Part model, mm, in its own coordinate system. A direction names the side the tool comes from. Give positions to 0.01 mm unless a question says otherwise; leave off trailing zeros. Order: outer loops, then holes, each group sorted by start corner. A loop starts at its lowest first (then second) coordinate and runs counter-clockwise, first axis right, second up.
1. Slice it at B-B on z = 36.5. List the corners of the cut face in (x, y) (3 decimals), and give its area (3 significant figures).
2. Drop flat-ended pins along their axis: pin 1 Ø11 at (x, y) = (5, 8) entering from +Z; pin 2 Ø6.5 at (x, y) = (24.5, 13.5) entering from +Z; pin 3 Ø1 at (x, z) = (-18, 8.5) entering from -Y. Give the stop position or say it passes through.
3. Probe line 1 (X direction, y = -8, z = 11); line 2 (Y direction, x = -13, z = 31); line 3 (X direction, y = 17.5, z = 23). List the from-to ranges inside material, lowest first.
4. Mould opens along X. For faces 1 (the flat face through (-4, 8, 25)), 2 (the flat face through (-35.965, -2.794, 25.832)), 3 (the flat face through (-38.5, 6, 15)) say: +X half, -X half, draft (parallel to the pull), parting line (faces both ways), or undercut.
5. Slice it at D-D on z = 4. List the corners of the cut face in (x, y).
6. Which spindle directions (+Z, -Z, +X, -X, +Y, -Y) get a long thin tool onto all of the face, cutting with end or side? Do faces 4 (the flat face through (22, 10, 35)), 5 (the flat face through (-16, 13, 20)), 6 (the flat face through (1.5, -19, 2)). Say none if no direction does.
7. Slice it at A-A on x = 6.5. List the corners of the cut face in (y, z), and give its area (3 significant figures).
8. Slice it at C-C on y = -18. List the corners of the cut face in (x, z).
from build123d import *

# Parameters (mm, degrees)
F0_W      = 35
F0_H      = 10
F1_DEPTH  = 5
F2_DEPTH  = 10
F3_DEPTH  = 15
F4_DEPTH  = 38
F5_DEPTH  = 38
F7_DEPTH  = 5
F8_DEPTH  = 15
F0_W_2    = 10
F0_H_2    = 22
F9_DEPTH  = 25
F10_DEPTH = 30
F11_DEPTH = 35
F12_DEPTH = 20
F0_W_3    = 5
F0_H_3    = 27
F13_DEPTH = 38


with BuildPart() as f1:
    # F0 (on Top) → F1 (new body)
    with BuildSketch(Plane.XY):
        with Locations((-16, -18.5)):
            Rectangle(F0_W, F0_H)
    extrude(amount=F1_DEPTH)

    # F0 (on Top) → F2 (join)
    with BuildSketch(Plane.XY):
        Polygon((33.5, -13.5), (33.5, -3.5), (11.5, -3.5), (1.5, -3.5), (-8.5, -3.5), (-33.5, -3.5), (-33.5, -13.5), (1.5, -13.5), align=None)
    extrude(amount=F2_DEPTH)

    # F0 (on Top) → F3 (join)
    with BuildSketch(Plane.XY):
        Polygon((38.5, -3.5), (33.5, -3.5), (33.5, -13.5), (33.5, -23.5), (38.5, -23.5), align=None)
    extrude(amount=F3_DEPTH)



with BuildPart() as f4:
    # F0 (on Top) → F4 (new body)
    with BuildSketch(Plane.XY):
        Polygon((11.5, 23.5), (-38.5, 23.5), (-38.5, 18.5), (-33.5, 18.5), (-8.5, 18.5), (1.5, 18.5), (11.5, 18.5), align=None)
    extrude(amount=F4_DEPTH)


with BuildPart() as f1_1:
    add(f1.part)

    add(f4.part)  # F5 merges F4
    # F0 (on Top) → F5 (join)
    with BuildSketch(Plane.XY):
        Polygon((-33.5, 18.5), (-38.5, 18.5), (-38.5, -23.5), (-33.5, -23.5), (-33.5, -13.5), (-33.5, -3.5), align=None)
    extrude(amount=F5_DEPTH)

    # F6 (on face) → F7 (cut)
    with BuildSketch(Plane.YZ.offset(-33.5)):
        Polygon((-23.5, 14), (18.5, 38), (-23.5, 38), align=None)
    extrude(amount=-F7_DEPTH, mode=Mode.SUBTRACT)

    # F0 (on Top) → F8 (join)
    with BuildSketch(Plane.XY):
        Polygon((-8.5, -3.5), (-33.5, 18.5), (-33.5, -3.5), align=None)
    extrude(amount=F8_DEPTH)

    # F0 (on Top) → F9 (join)
    with BuildSketch(Plane.XY):
        with Locations((-3.5, 7.5)):
            Rectangle(F0_W_2, F0_H_2)
    extrude(amount=F9_DEPTH)

    # F0 (on Top) → F10 (join)
    with BuildSketch(Plane.XY):
        with Locations((6.5, 7.5)):
            Rectangle(F0_W_2, F0_H_2)
    extrude(amount=F10_DEPTH)

    # F0 (on Top) → F11 (join)
    with BuildSketch(Plane.XY):
        Polygon((33.5, 23.5), (11.5, 23.5), (11.5, 18.5), (11.5, -3.5), (33.5, -3.5), align=None)
    extrude(amount=F11_DEPTH)

    # F0 (on Top) → F12 (join)
    with BuildSketch(Plane.XY):
        Polygon((-8.5, 18.5), (-33.5, 18.5), (-8.5, -3.5), align=None)
    extrude(amount=F12_DEPTH)

    # F0 (on Top) → F13 (join)
    with BuildSketch(Plane.XY):
        with Locations((36, 10)):
            Rectangle(F0_W_3, F0_H_3)
    extrude(amount=F13_DEPTH)


solid = f1_1.part
Data:
1. outline: (-38.5, 15.875) - (-33.5, 15.875) - (-33.5, 18.5) - (11.5, 18.5) - (11.5, 23.5) - (-38.5, 23.5) - close; (33.5, -3.5) - (38.5, -3.5) - (38.5, 23.5) - (33.5, 23.5) - close
1. area: 398 mm2
2. pin 1: stops at z = 30
2. pin 2: stops at z = 35
2. pin 3: stops at y = -13.5
3. line 1: x = -38.5 to -33.5, 33.5 to 38.5
3. line 2: y = 18.5 to 23.5
3. line 3: x = -38.5 to -33.5, -8.5 to 38.5
4. face 1: undercut
4. face 2: draft
4. face 3: -X half
5. outline: (-38.5, -23.5) - (1.5, -23.5) - (1.5, -13.5) - (33.5, -13.5) - (33.5, -23.5) - (38.5, -23.5) - (38.5, 23.5) - (-38.5, 23.5) - close
6. face 4: +Z, +Y, -Y
6. face 5: +Z, -Y
6. face 6: +Z, -Z, -Y
7. outline: (-13.5, 0) - (23.5, 0) - (23.5, 38) - (18.5, 38) - (18.5, 30) - (-3.5, 30) - (-3.5, 10) - (-13.5, 10) - close
7. area: 950 mm2
8. outline: (-38.5, 0) - (1.5, 0) - (1.5, 5) - (-33.5, 5) - (-33.5, 17.14) - (-38.5, 17.14) - close; (33.5, 0) - (38.5, 0) - (38.5, 15) - (33.5, 15) - close
